Source: CAD feature listing. Evaluate the final solid. Frame: model axes, mm. Give positions to 0.01 mm unless a question says otherwise; leave off trailing zeros.
from build123d import *

# Parameters (mm, degrees)
SKETCH1_R           = 2.5
BOSS_EXTRUDE1_DEPTH = 240


with BuildPart() as part:
    # Sketch1 → Boss-Extrude1 (new, symmetric)
    with BuildSketch(Plane(origin=(0, 0, 0), x_dir=(1, 0, 0), z_dir=(0, 1, 0))):
        with BuildLine():
            Line((-7, -10), (-7, -8))
            Line((-7, -8), (-4.5, -8))
            Line((-4.5, -8), (-4.5, -6.914213562))
            Line((-4.5, -6.914213562), (-7.814213562, -3.6))
            Line((-7.814213562, -3.6), (-12.185786438, -3.6))
            Line((-12.185786438, -3.6), (-15.5, -6.914213562))
            Line((-15.5, -6.914213562), (-15.5, -8))
            Line((-15.5, -8), (-13, -8))
            Line((-13, -8), (-13, -10))
            Line((-13, -10), (-18.5, -10))
            ThreePointArc((-18.5, -10), (-19.560660172, -9.560660172), (-20, -8.5))
            Line((-20, -8.5), (-20, -3))
            Line((-20, -3), (-18, -3))
            Line((-18, -3), (-18, -5.5))
            Line((-18, -5.5), (-16.914213562, -5.5))
            Line((-16.914213562, -5.5), (-13.6, -2.185786438))
            Line((-13.6, -2.185786438), (-13.6, 2.185786438))
            Line((-13.6, 2.185786438), (-16.914213562, 5.5))
            Line((-16.914213562, 5.5), (-18, 5.5))
            Line((-18, 5.5), (-18, 3))
            Line((-18, 3), (-20, 3))
            Line((-20, 3), (-20, 8.5))
            ThreePointArc((-20, 8.5), (-19.560660172, 9.560660172), (-18.5, 10))
            Line((-18.5, 10), (-13, 10))
            Line((-13, 10), (-13, 8))
            Line((-13, 8), (-15.5, 8))
            Line((-15.5, 8), (-15.5, 6.914213562))
            Line((-15.5, 6.914213562), (-12.185786438, 3.6))
            Line((-12.185786438, 3.6), (-7.814213562, 3.6))
            Line((-7.814213562, 3.6), (-4.5, 6.914213562))
            Line((-4.5, 6.914213562), (-4.5, 8))
            Line((-4.5, 8), (-7, 8))
            Line((-7, 8), (-7, 10))
            Line((-7, 10), (7, 10))
            Line((7, 10), (7, 8))
            Line((7, 8), (4.5, 8))
            Line((4.5, 8), (4.5, 6.914213562))
            Line((4.5, 6.914213562), (7.814213562, 3.6))
            Line((7.814213562, 3.6), (12.185786438, 3.6))
            Line((12.185786438, 3.6), (15.5, 6.914213562))
            Line((15.5, 6.914213562), (15.5, 8))
            Line((15.5, 8), (13, 8))
            Line((13, 8), (13, 10))
            Line((13, 10), (18.5, 10))
            ThreePointArc((18.5, 10), (19.560660172, 9.560660172), (20, 8.5))
            Line((20, 8.5), (20, 3))
            Line((20, 3), (18, 3))
            Line((18, 3), (18, 5.5))
            Line((18, 5.5), (16.914213562, 5.5))
            Line((16.914213562, 5.5), (13.6, 2.185786438))
            Line((13.6, 2.185786438), (13.6, -2.185786438))
            Line((13.6, -2.185786438), (16.914213562, -5.5))
            Line((16.914213562, -5.5), (18, -5.5))
            Line((18, -5.5), (18, -3))
            Line((18, -3), (20, -3))
            Line((20, -3), (20, -8.5))
            ThreePointArc((20, -8.5), (19.560660172, -9.560660172), (18.5, -10))
            Line((18.5, -10), (13, -10))
            Line((13, -10), (13, -8))
            Line((13, -8), (15.5, -8))
            Line((15.5, -8), (15.5, -6.914213562))
            Line((15.5, -6.914213562), (12.185786438, -3.6))
            Line((12.185786438, -3.6), (7.814213562, -3.6))
            Line((7.814213562, -3.6), (4.5, -6.914213562))
            Line((4.5, -6.914213562), (4.5, -8))
            Line((4.5, -8), (7, -8))
            Line((7, -8), (7, -10))
            Line((7, -10), (-7, -10))
        make_face()
        with Locations(Location((-10, 0, 0), (0, 0, 90))):
            Circle(SKETCH1_R, mode=Mode.SUBTRACT)
        with Locations(Location((10, 0, 0), (0, 0, 270))):
            Circle(SKETCH1_R, mode=Mode.SUBTRACT)
        Polygon((-2.5, 8), (-2.5, 6.085786438), (-6.4, 2.185786438), (-6.4, -2.185786438), (-2.5, -6.085786438), (-2.5, -8), (2.5, -8), (2.5, -6.085786438), (6.4, -2.185786438), (6.4, 2.185786438), (2.5, 6.085786438), (2.5, 8), align=None, mode=Mode.SUBTRACT)
    extrude(amount=BOSS_EXTRUDE1_DEPTH, both=True)


solid = part.part
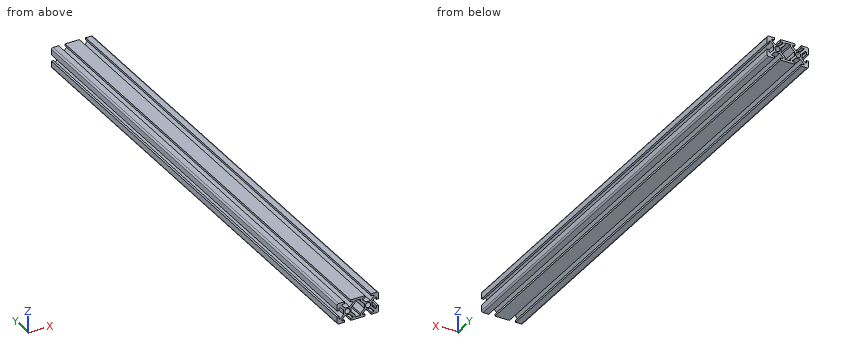
(1) Line query: line 1 along X through (y, z) = (-109.5, -8.75); line 2 along Z through (x, y) = (5, -200.5); line 3 along X through (y, z) = (66.5, 0). Output: solid intervals per line, ascending.
(2) Pin query (flat end, axial travel): pin 1 Ø5 at (y, z) = (22, 0) entering from +X; pin 2 Ø1.6 at (y, z) = (71.5, -9.5) entering from -X; pin 3 Ø2 at (x, y) = (-10, -77.5) entering from +Z. Return the tip coordinate at first contact, or that it passes through.
(3) Section A-A, the plane y = -177. Count the separate pieces of the cut face and the enclosed holes in it, plus the area to 3 significant figures.
Checks:
1. line 1: x = -19.98 to -13, -7 to 7, 13 to 19.98
1. line 2: z = -10 to -8, -6.41 to -3.59, 3.59 to 6.41, 8 to 10
1. line 3: x = -13.6 to -12.5, -7.5 to -6.4, 6.4 to 7.5, 12.5 to 13.6
2. pin 1: stops at x = 13.91
2. pin 2: stops at x = -19.99
2. pin 3: stops at z = 3.6
3. separate pieces: 1
3. enclosed holes: 3
3. area: 318 mm2
